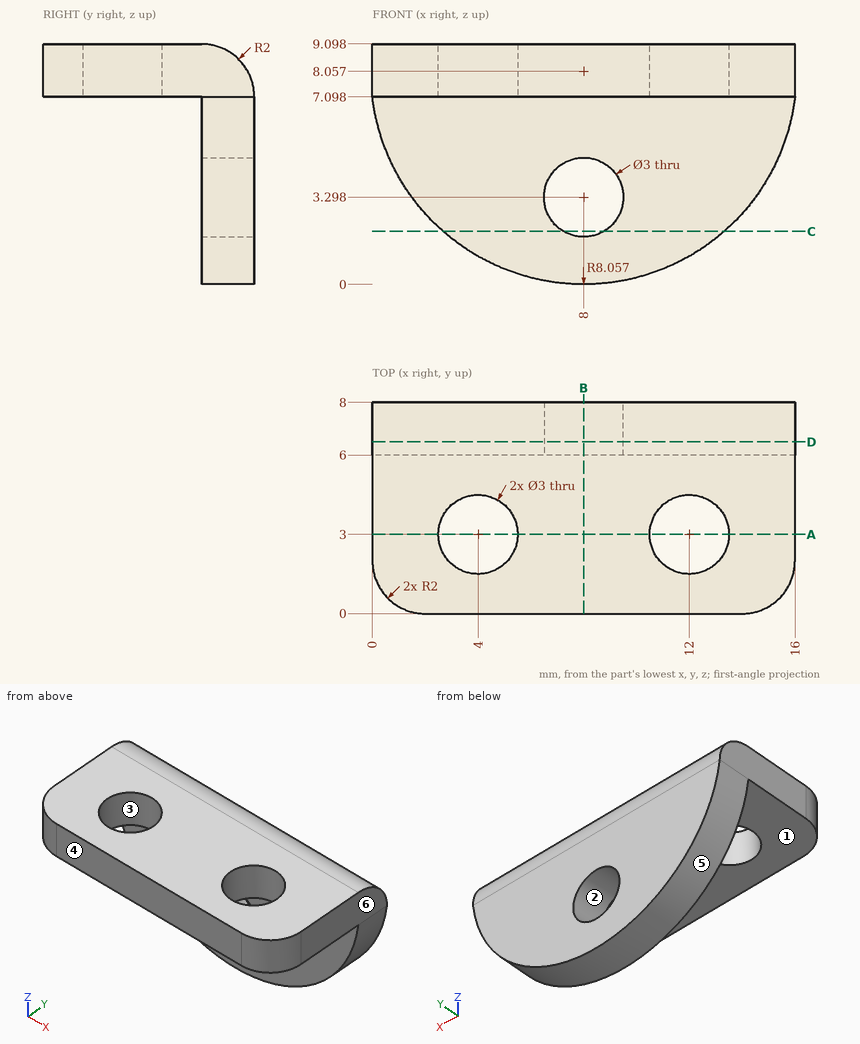
Check sheet for the drawn part. Datum: minimum x, y, z corner. Units: mm. A direction names the side the tool comes from. Round coordinates to 2 decimals unless told otherwise and drop trailing zeros. Order: outer loops, then holes, each group sorted by start corner. A loop starts at its lowest first (then second) coordinate and runs counter-clockwise, first axis right, second up. Notation, with made-up numbers: (21.25, 65.5) -> (44.25, 65.5) arc R15 cw to (44.25, 91.5) -> close; hole circle Ø3 at (89, -24). An arc over 180 degrees is marked (long way). Use CSV: the item, a comma, the result in double quotes.
(1) Draft check along X on the marked faces 3, 4, 5 and 6. Enter one of: pulls with the +X half, pulls with the -X half, needs draft (parallel to the pull), parting line crosses it, or undercut.
Worked out:
face 3,"undercut"
face 4,"needs draft"
face 5,"parting line crosses it"
face 6,"pulls with the +X half"
(2) Cross-section at A-A (y = 3). Record the boundary of the cut face in (x, z), and give its area (3 significant figures).
Worked out:
outline,"(0, 7.1) -> (2.5, 7.1) -> (2.5, 9.1) -> (0, 9.1) -> close; (5.5, 7.1) -> (10.5, 7.1) -> (10.5, 9.1) -> (5.5, 9.1) -> close; (13.5, 7.1) -> (16, 7.1) -> (16, 9.1) -> (13.5, 9.1) -> close"
area,"20.0 mm²"
(3) Tool access check on the marked faces 1 and 2. Record the directions out of +Z, -Z, +X, -X, +Y, -Y that give a thin tool (end or side, any length) a straight path to the whole face; none if there is none.
Worked out:
face 1,"-Z, +X, -X, -Y"
face 2,"+Y, -Y"
(4) Depth check by flat-ended pin: pin 1 (1 mm diameter, centred on y = 4, z = 3.5, fed in from +X); pin 2 (4 mm diameter, centred on x = 6, y = 3.5, fed in from -Z); pin 3 (3.5 mm diameter, centred on x = 4, y = 3, fed in from +Z); pin 4 (1.5 mm diameter, centred on x = 6, z = 5, fed in from -Y). Enter the tip coordinate at first touch or a pass-through.
Worked out:
pin 1,"through"
pin 2,"z = 7.1"
pin 3,"z = 9.1"
pin 4,"y = 6"
(5) Cross-section at B-B (x = 8). Record the boundary of the cut face in (y, z).
Worked out:
outline,"(0, 7.1) -> (6, 7.1) -> (6, 4.8) -> (8, 4.8) -> (8, 7.1) arc R2 ccw to (6, 9.1) -> (0, 9.1) -> close; (6, 0) -> (8, 0) -> (8, 1.8) -> (6, 1.8) -> close"
(6) Cross-section at D-D (y = 6.5). Record the boundary of the cut face in (x, z) (1 decimal).
Worked out:
outline,"(0, 7.1) arc R8.1 ccw to (16, 7.1) -> (16, 9) -> (0, 9) -> close; hole circle Ø3 at (8, 3.3)"
(7) Cross-section at C-C (z = 2). Record the boundary of the cut face in (x, y).
Worked out:
outline,"(2.69, 6) -> (7.25, 6) -> (7.25, 8) -> (2.69, 8) -> close; (8.75, 6) -> (13.31, 6) -> (13.31, 8) -> (8.75, 8) -> close"
(8) Material ranges on line 1 along Z through (x, y) = (6.75, 3); line 2 along Y through (x, z) = (4.5, 4); line 3 along X through (y, z) = (2.25, 8), recorded low to high. Write a range as from..to.
Worked out:
line 1,"7.1..9.1"
line 2,"6..8"
line 3,"0..2.7, 5.3..10.7, 13.3..16"
